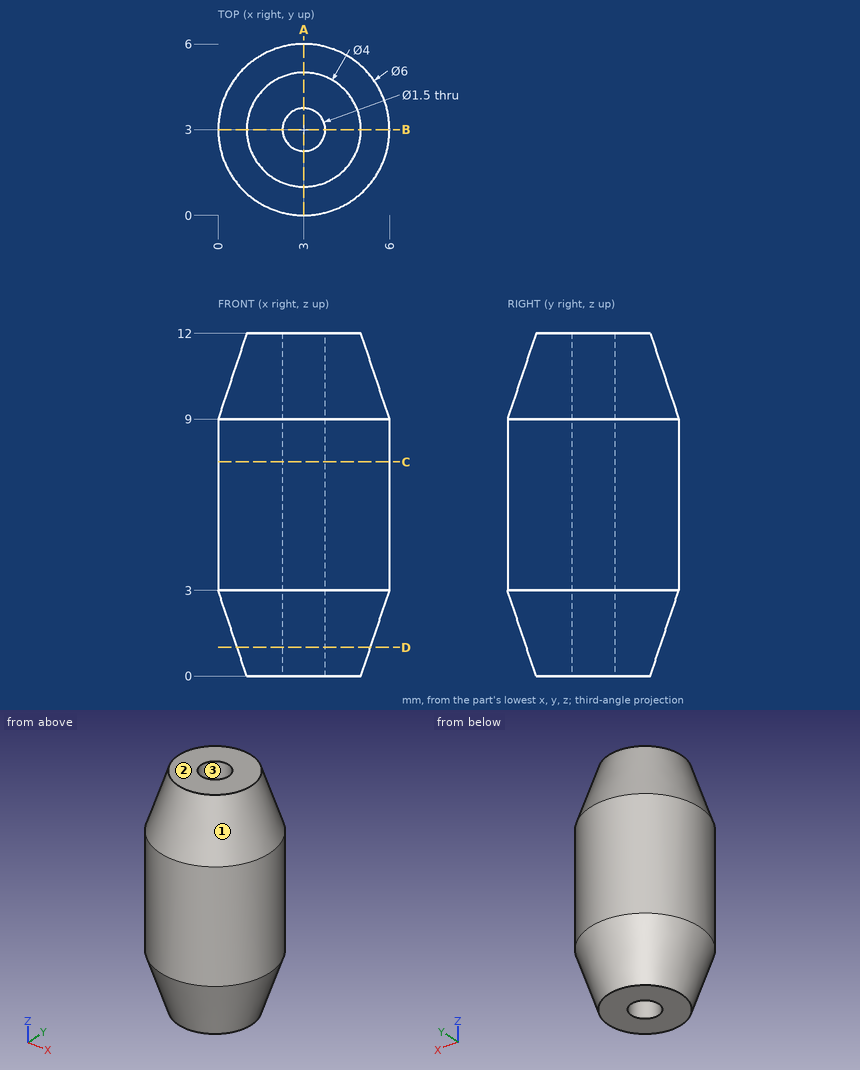
Verification items for this drawing (mm, ordinates from the low corner). Coordinates: 2 decimals unless noted, no trailing zeros. Loops run counter-clockwise (first coordinate to the right, second up) from the corner with the lowest first, then second, coordinate; pieces in that order, holes last. Notation, with made-up numbers: (37, 68.5) - (78, 68.5) arc R19 ccw to (78, 86.5) - close; hole circle Ø10 at (61.25, -8.5). An arc over 180 degrees is marked (long way). Answer as a JSON object with one key per item and string values.
(1) Mould release check, pull along Y, two halves, no side actions. Record for the marked faces 1, 2 and 3: pulls with the +Y half, pulls with the -Y half, needs draft (parallel to the pull), parting line crosses it, or undercut.
Response:
{"face 1": "parting line crosses it", "face 2": "needs draft", "face 3": "undercut"}
(2) Scan lines: line 1 along Y through (x, z) = (3, 8.75); line 2 along Y through (x, z) = (2.6, 6.75); line 3 along X through (y, z) = (3.35, 5.5). Record each from-to range of solid material in increasing order.
Response:
{"line 1": "y = 0 to 2.25, 3.75 to 6", "line 2": "y = 0.03 to 2.37, 3.63 to 5.97", "line 3": "x = 0.02 to 2.34, 3.66 to 5.98"}
(3) Cross-section at D-D, the plane z = 1. Record the boundary of the cut face in (x, y).
Response:
{"outline": "circle Ø4.67 at (3, 3); hole circle Ø1.5 at (3, 3)"}
(4) Cross-section at A-A, the plane x = 3. Record the boundary of the cut face in (y, z).
Response:
{"outline": "(0, 3) - (1, 0) - (2.25, 0) - (2.25, 12) - (1, 12) - (0, 9) - close; (3.75, 0) - (5, 0) - (6, 3) - (6, 9) - (5, 12) - (3.75, 12) - close"}
(5) Cross-section at C-C, the plane z = 7.5. Record the boundary of the cut face in (x, y), then the cut area to 3 significant figures.
Response:
{"outline": "circle Ø6 at (3, 3); hole circle Ø1.5 at (3, 3)", "area": "26.5 mm²"}
